For this review, use the dimensioned drawing (mm, ordinates from the lowest corner) and the shaded views. Coordinates: 2 decimals unless noted, no trailing zeros. Order: outer loops, then holes, each group sorted by start corner. A loop starts at its lowest first (then second) coordinate and runs counter-clockwise, first axis right, second up. Notation, with made-up numbers: M 59.25,75.25 L 71.25,75.25 A12 ccw 71.25,80.25 Z; hole C 66,32.25 d2. An arc over 180 degrees is marked long. Write each question's results on one line, items separated by ' | '.
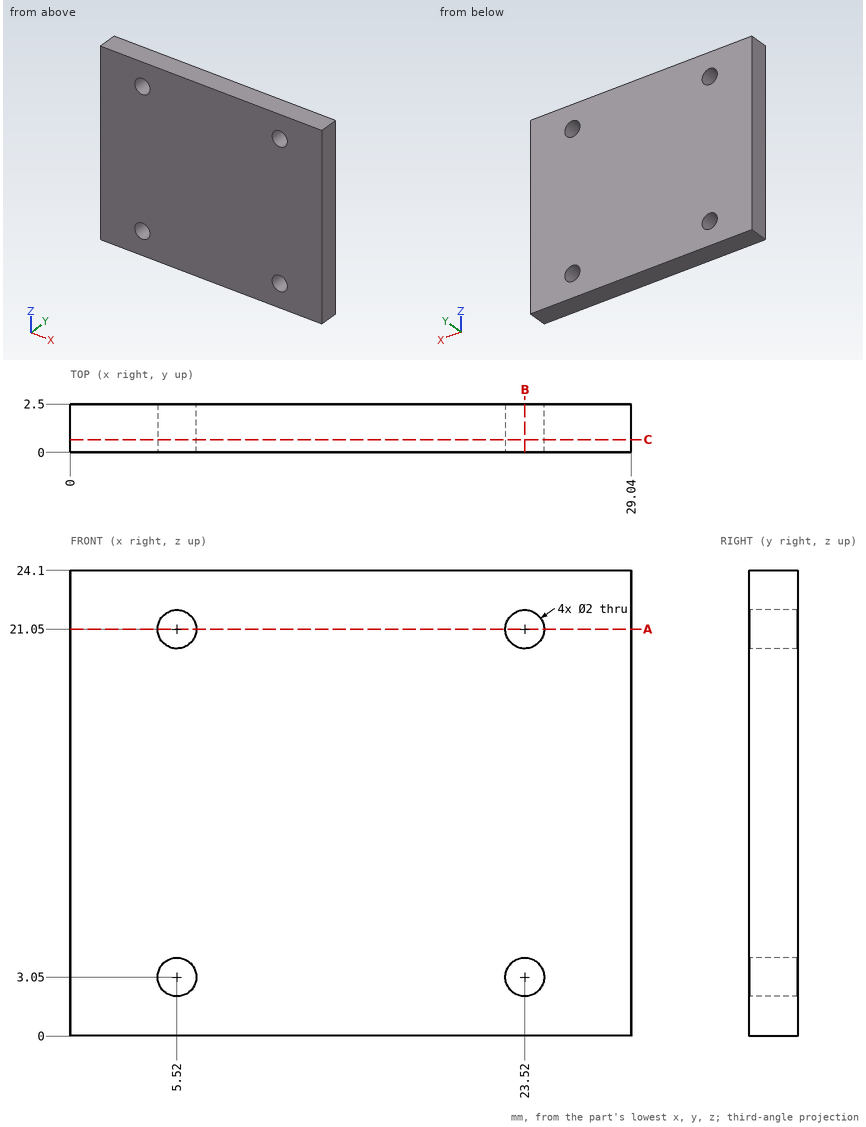
1) Take a section at A-A on z = 21.05. State the section outline as (x, y) points, plus the area to 3 significant figures.
Solutions:
outline: M 0,0 L 4.52,0 L 4.52,2.5 L 0,2.5 Z; M 6.52,0 L 22.52,0 L 22.52,2.5 L 6.52,2.5 Z; M 24.52,0 L 29.04,0 L 29.04,2.5 L 24.52,2.5 Z | area: 62.6 mm2
2) For pin 1 (3 mm diameter, centred on x = 5.52, z = 3.05, fed in from +Y), flat-tipped, find the tip position at first contact; note if it passes through.
Solutions:
pin 1: y = 2.5
3) Take a section at C-C on y = 0.65. State the section outline as (x, z) points, plus the area to 3 significant figures.
Solutions:
outline: M 0,0 L 29.04,0 L 29.04,24.1 L 0,24.1 Z; hole C 5.52,3.05 d2; hole C 5.52,21.05 d2; hole C 23.52,3.05 d2; hole C 23.52,21.05 d2 | area: 687 mm2
4) To check wall thickness, follow line 1 along Z through (x, y) = (23.5, 2.4); line 2 along X through (y, z) = (1.4, 21.05); line 3 along Z through (x, y) = (4.75, 0.9). State the ranges of each line that lie inside material, in increasing order.
Solutions:
line 1: 0 to 2.05, 4.05 to 20.05, 22.05 to 24.1 | line 2: 0 to 4.52, 6.52 to 22.52, 24.52 to 29.04 | line 3: 0 to 2.41, 3.69 to 20.41, 21.69 to 24.1
5) Take a section at B-B on x = 23.52. State the section outline as (y, z) points, plus the area to 4 significant figures.
Solutions:
outline: M 0,0 L 2.5,0 L 2.5,2.05 L 0,2.05 Z; M 0,4.05 L 2.5,4.05 L 2.5,20.05 L 0,20.05 Z; M 0,22.05 L 2.5,22.05 L 2.5,24.1 L 0,24.1 Z | area: 50.25 mm2
